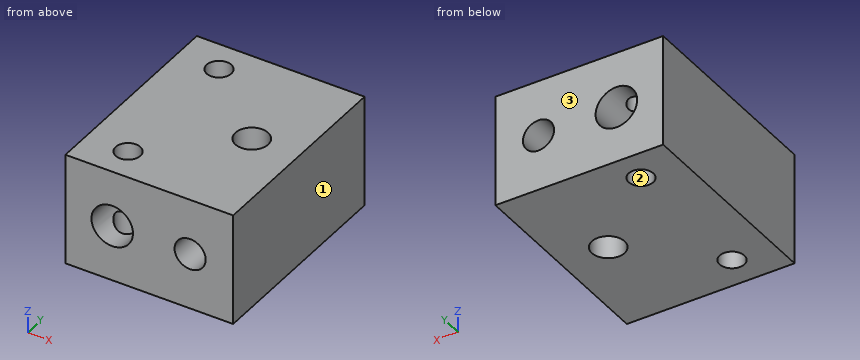
from build123d import *

# Parameters (mm, degrees)
SKETCH1_W           = 21
SKETCH1_H           = 14
BOSS_EXTRUDE2_DEPTH = 26
CUT_EXTRUDE1_DEPTH  = 26
CUT_EXTRUDE2_DEPTH  = 26


with BuildPart() as part:
    # Sketch1 → Boss-Extrude2 (new body)
    with BuildSketch(Plane(origin=(0, 0, 0), x_dir=(1, 0, 0), z_dir=(0, 1, 0))):
        Rectangle(SKETCH1_W, SKETCH1_H)
    extrude(amount=BOSS_EXTRUDE2_DEPTH)

    # Sketch3 → Cut-Extrude1 (cut)
    with BuildSketch(Plane.XY.offset(7)):
        with BuildLine():
            ThreePointArc((-3.687132732, 4.065349549), (-5.237132732, 5.615349549), (-6.787132732, 4.065349549))
            ThreePointArc((-6.787132732, 4.065349549), (-5.237132732, 2.515349549), (-3.687132732, 4.065349549))
        make_face()
        with BuildLine():
            ThreePointArc((6.612867268, 13.065349549), (4.562867268, 15.115349549), (2.512867268, 13.065349549))
            ThreePointArc((2.512867268, 13.065349549), (4.562867268, 11.015349549), (6.612867268, 13.065349549))
        make_face()
        with BuildLine():
            ThreePointArc((-3.687132732, 22.065349549), (-5.237132732, 23.615349549), (-6.787132732, 22.065349549))
            ThreePointArc((-6.787132732, 22.065349549), (-5.237132732, 20.515349549), (-3.687132732, 22.065349549))
        make_face()
    extrude(amount=-CUT_EXTRUDE1_DEPTH, mode=Mode.SUBTRACT)

    # Sketch4 → Cut-Extrude2 (cut)
    with BuildSketch(Plane(origin=(0, 26, 0), x_dir=(1, 0, 0), z_dir=(0, 1, 0))):
        with BuildLine():
            ThreePointArc((-2.040636321, 0), (-4.640636321, 2.6), (-7.240636321, 0))
            ThreePointArc((-7.240636321, 0), (-4.640636321, -2.6), (-2.040636321, 0))
        make_face()
        with BuildLine():
            ThreePointArc((3.159363679, 0), (5.109363679, -1.95), (7.059363679, 0))
            ThreePointArc((7.059363679, 0), (5.109363679, 1.95), (3.159363679, 0))
        make_face()
    extrude(amount=-CUT_EXTRUDE2_DEPTH, mode=Mode.SUBTRACT)


solid = part.part
Could you check a few things on this model? Use its own coordinates, in mm. Face numbers are marked on the shaded views. Give positions to 0.01 mm unless a question says otherwise; leave off trailing zeros. Order: outer loops, then holes, each group sorted by start corner. A loop starts at its lowest first (then second) coordinate and runs counter-clockwise, first axis right, second up.
1. Suppose I cut it at A-A (y = 4.5). List the corners of the cut face in (x, z) for me, plus the area to 3 significant figures.
2. We'd pull the mould along Y, two halves only. Please class the marked faces 1, 2 and 3: pulls with the +Y half, pulls with the -Y half, needs draft (parallel to the pull), parting line crosses it, or undercut.
3. Suppose I cut it at D-D (y = 10.5). List the corners of the cut face in (x, z) for me.
4. I need wall thicknesses on L1, parallel to Z at x = 5.25, y = 6.75; L2, parallel to X at y = 12.5, z = 1.5; L3, parallel to X at y = 5.5, z = 1. Which ranges of each line are inside material? Lowest first, please.
5. Suppose I cut it at B-B (z = 0). List the corners of the cut face in (x, y) for me, plus the area to 3 significant figures.
6. Suppose I cut it at C-C (z = 4.75). List the corners of the cut face in (x, y) for me.
Solved:
1. outline: (-10.5, -7) - (-6.72, -7) - (-6.72, -1.55) arc R2.6 cw to (-6.72, 1.55) - (-6.72, 7) - (-10.5, 7) - close; (-3.75, -7) - (10.5, -7) - (10.5, 7) - (-3.75, 7) - (-3.75, 2.44) arc R2.6 cw to (-3.75, -2.44) - close; hole circle Ø3.9 at (5.11, 0)
1. area: 233 mm2
2. face 1: needs draft
2. face 2: undercut
2. face 3: pulls with the +Y half
3. outline: (-10.5, -7) - (10.5, -7) - (10.5, 7) - (-10.5, 7) - close; hole circle Ø5.2 at (-4.64, 0); hole circle Ø3.9 at (5.11, 0)
4. L1: z = -7 to -1.94, 1.94 to 7
4. L2: x = -10.5 to -6.76, -2.52 to 2.59, 6.53 to 10.5
4. L3: x = -10.5 to -7.04, -2.24 to 3.44, 6.78 to 10.5
5. outline: (-10.5, 0) - (-7.24, 0) - (-7.24, 26) - (-10.5, 26) - close; (-2.04, 0) - (3.16, 0) - (3.16, 11.57) arc R2.05 cw to (3.16, 14.56) - (3.16, 26) - (-2.04, 26) - close; (7.06, 0) - (10.5, 0) - (10.5, 26) - (7.06, 26) - close
5. area: 308 mm2
6. outline: (-10.5, 0) - (10.5, 0) - (10.5, 26) - (-10.5, 26) - close; hole circle Ø3.1 at (-5.24, 4.07); hole circle Ø3.1 at (-5.24, 22.07); hole circle Ø4.1 at (4.56, 13.07)
